Autodesk Inventor part; units mm, degrees
ref_plane "YZ Plane" through (0, 0, 0) normal (1, 0, 0) x (0, 1, 0)
ref_plane "XZ Plane" through (0, 0, 0) normal (0, 1, 0) x (-1, 0, 0)
ref_plane "XY Plane" through (0, 0, 0) normal (0, 0, 1) x (1, 0, 0)
sketch "Szkic2" plane through (0, 0, 0) normal (0, 1, 0) x (-1, 0, 0)
  line L0 (-6, 6) -> (6, 6)
  line L1 (6, 6) -> (6, -6)
  line L2 (6, -6) -> (-6, -6)
  line L3 (-6, -6) -> (-6, 6)
  line L4 (-6, 6) -> (6, -6) construction
  line L5 (6, 6) -> (-6, -6) construction
  point P0 (0, 0)
  dimension "d3" = 12
  dimension "d4" = 12
extrude "Wyciągnięcie proste1" add sketch "Szkic2" along normal blind 8
sketch "Szkic5" plane through (-6, 0, -6) normal (-1, 0, 0) x (0, 0, 1)
  line L0 (0, 8) -> (12, 8)
  line L1 (6, 8) -> (6, 0)
  line L2 (6, 0) -> (6, 8)
  line L3 (6, 8) -> (6, 4)
  circle A0 centre (6, 4) radius 1.5
  dimension "d10" = 4
  dimension "d11" = 3
extrude "Wyciągnięcie proste2" cut sketch "Szkic5" against normal through all
thread "Gwint1"
sketch "Szkic6" plane through (0, 0, 0) normal (0, -1, 0) x (1, 0, 0)
  circle A0 centre (0, 0) radius 6
  circle A1 centre (0, 0) radius 8
  circle A2 centre (0, 0) radius 2
  line L0 (0, 0) -> (2, 0)
  line L1 (0, 0) -> (-1.6, 0)
  line L2 (-1.6, 0) -> (-1.6, -1.2)
  line L3 (-1.6, 0) -> (-1.6, 1.2)
  line L4 (-6, 6) -> (6, 6)
  circle A3 centre (0, 0) radius 8.4853
  point P0 (-5.2915, 6)
  point P1 (5.2915, 6)
  point P2 (0, 6)
extrude "Wyciągnięcie proste3" cut sketch "Szkic6" against normal blind 8 contours L4 A1 | L4 A3 A1 | A1 L4 A3 | L0 L1 L3 A2 | A2 L2 L1 L0 picked at (7.1897, -1.149)
sketch "Szkic11" plane through (0, 0, 0) normal (0, -1, 0) x (1, 0, 0)
  circle A0 centre (0, 0) radius 6
  circle A1 centre (0, 0) radius 7
  dimension "d24" = 14
extrude "Wyciągnięcie proste4" add sketch "Szkic11" along normal blind 12 contours A0 | A1
sketch "Szkic18" plane through (0, -12, 0) normal (0, -1, 0) x (1, 0, 0)
  arc A0 (-1.6, -1.2) -> (-1.6, 1.2) centre (0, 0) ccw
  circle A1 centre (0, 0) radius 12.5
  dimension "d35" = 25
loft "Wyciągnięcie złożone2" add profiles "Szkic18" section 2 edges at (0, 0, -6)
sketch "Szkic19" plane through (0, -12, 0) normal (0, -1, 0) x (1, 0, 0)
  circle A0 centre (0, 0) radius 12.5
sketch "Szkic20" plane through (0, -12, 0) normal (0, -1, 0) x (1, 0, 0)
  point P0 (0, 0)
extrude "Wyciągnięcie proste6" add sketch "Szkic19" along normal blind 5
sketch "Szkic21" plane through (0, -17, 0) normal (0, -1, 0) x (1, 0, 0)
  line L0 (-11, 11) -> (11, 11)
  line L1 (11, 11) -> (11, -11)
  line L2 (11, -11) -> (-11, -11)
  line L3 (-11, -11) -> (-11, 11)
  circle A0 centre (0, 0) radius 6
  line L4 (-11, 11) -> (11, -11) construction
  line L5 (11, 11) -> (-11, -11) construction
  circle A1 centre (0, 0) radius 12.5
  point P0 (5.9372, 11)
  point P1 (-5.9372, 11)
  point P2 (11, 5.9372)
  point P3 (11, -5.9372)
  point P4 (-11, 5.9372)
  point P5 (-11, -5.9372)
  point P6 (-5.9372, -11)
  point P7 (5.9372, -11)
  dimension "d42" = 22
  dimension "d43" = 22
extrude "Wyciągnięcie proste7" cut sketch "Szkic21" against normal through all contours A1 L0 | L3 A1 | A1 L1 | L2 A1
sketch "Szkic22" plane through (0, -17, 0) normal (0, -1, 0) x (1, 0, 0)
  line L0 (0, 0) -> (-7, 0)
  line L1 (0, 0) -> (7, 0)
  circle A0 centre (-7, 0) radius 1.5
  circle A1 centre (7, 0) radius 1.5
  dimension "d46" = 7
  dimension "d47" = 7
  dimension "d48" = 3
  dimension "d49" = 3
extrude "Wyciągnięcie proste8" cut sketch "Szkic22" against normal blind 5
thread "Gwint2"
thread "Gwint3"
fillet "Zaokrąglenie1" radius 2.2 1 edges at (-7, 0, 0)
properties part number "MocowanieChwytakaElement1"
The listing builds one solid part. Answer for the finished solid, in the listing's coordinates (mm). A direction names the side the tool comes from. Coordinates: 2 decimals unless noted, no trailing zeros. Loops run counter-clockwise (first coordinate to the right, second up) from the corner with the lowest first, then second, coordinate; pieces in that order, holes last. Notation, with made-up numbers: M 24.25,-39 L 36.25,-39 A22 ccw 36.25,-6 Z; hole C 36.25,36 d5. An arc over 180 degrees is marked long. Answer in a Markdown table with one row per item.
1) Find section C-C (y = -14). Determine the outline of the cut face in (x, z), then the cut area to 3 significant figures.
Answers below:
| item | result |
|---|---|
| outline | M -11,-5.94 A12.5 ccw -5.94,-11 L 5.94,-11 A12.5 ccw 11,-5.94 L 11,5.94 A12.5 ccw 5.94,11 L -5.94,11 A12.5 ccw -11,5.94 Z; hole C -7,0 d3; hole C 7,0 d3 |
| area | 429 mm^2 |
2) Find section D-D (z = 0). Count the separate pieces of the cut face and the enclosed holes in it, then the cut area to 3 significant figures.
Answers below:
| item | result |
|---|---|
| separate pieces | 3 |
| enclosed holes | 0 |
| area | 341 mm^2 |
3) Find the intervals of material crossed by probe 1 along Y at (x, z) = (3.05, 0); probe 2 along Z at (x, y) = (4, 5.25); probe 3 along Y at (x, z) = (-9, 0), in increasing order.
Answers below:
| item | result |
|---|---|
| probe 1 | -17 to 2.5, 5.5 to 8 |
| probe 2 | -4.47 to -0.83, 0.83 to 4.47 |
| probe 3 | -17 to -5.54 |
4) Given pin 1 (1.8 mm diameter, centred on y = 4, z = 0, fed in from -X) (1 decimal); pin 2 (4 mm diameter, centred on y = -3.5, z = -8.5, fed in from +X); pin 3 (4 mm diameter, centred on y = 1.5, z = 6, fed in from -X); pin 4 (2.5 mm diameter, centred on x = 7, z = 0, fed in from -Y), each flat-ended and moving along its own axis, determine where each tip first touches the part or whether it passes through.
Answers below:
| item | result |
|---|---|
| pin 1 | through |
| pin 2 | x = 5.05 |
| pin 3 | x = -4.47 |
| pin 4 | y = -12 |
5) Determine the mould class of faces 1 (the cylindrical face through (0.95, 3.94, 1.76)), 2 (the conical face through (6.8, -2.5, -2.8)), 3 (the flat face through (-3, 8, 0)) for opening direction X: released by +X, released by -X, zero draft, split by the parting line, or undercut.
Answers below:
| item | result |
|---|---|
| face 1 | undercut |
| face 2 | split by the parting line |
| face 3 | zero draft |
6) Which of the six approach directions +Z, -Z, +X, -X, +Y, -Y give full straight-line access (tool end or side, diameter ignored) to faces 4 (the flat face through (-1.6, 7, 0)), 5 (the flat face through (0, -13, -11)), 6 (the flat face through (7, -12, 0))?
Answers below:
| item | result |
|---|---|
| face 4 | +Y |
| face 5 | -Z, +X, -X, +Y, -Y |
| face 6 | -Y |
7) Find section A-A (y = 4). Determine the outline of the cut face in (x, z).
Answers below:
| item | result |
|---|---|
| outline | M -5.81,-1.5 A6 ccw 5.81,-1.5 L 1.32,-1.5 A2 cw -1.32,-1.5 Z; M -5.81,1.5 L -1.32,1.5 A2 cw 1.32,1.5 L 5.81,1.5 A6 ccw Z |
